Geometry: see drawing. Coordinates: mm, zero at the bounding-box minimum. Round coordinates to 2 decimals unless told otherwise and drop trailing zeros. Loops run counter-clockwise (first coordinate to the right, second up) from the corner with the lowest first, then second, coordinate; pieces in that order, holes last.
(1) Section C-C, the plane y = 14.5. Return the cut outline in (x, z), plus the area to 3 significant figures.
(2) Section A-A, the plane x = 33.5. Return the cut outline in (y, z).
(3) Section B-B, the plane z = 33.5. Return the cut outline in (x, y), plus the area to 3 significant figures.
(4) Material intervals for probe 1 along Z at (x, y) = (33.5, 17.75); probe 2 along Z at (x, y) = (45, 17); probe 3 along X at (y, z) = (18.75, 16.5), sorted ascending.
(5) Mould query, pull axis Z, two halves, no side actions, for the marked faces 1 and 2. Classes: pulls with the +Z half, pulls with the -Z half, needs draft (parallel to the pull), parting line crosses it, or undercut.
(6) First-contact query: pin 1 Ø6 at (y, z) = (7, 51.5) entering from -X; pin 2 Ø5 at (y, z) = (14.5, 43) entering from +X; pin 3 Ø8 at (x, y) = (18, 14.5) entering from -Z. Flat tips, straight axial feed; report the tip coordinate or a pass-through.
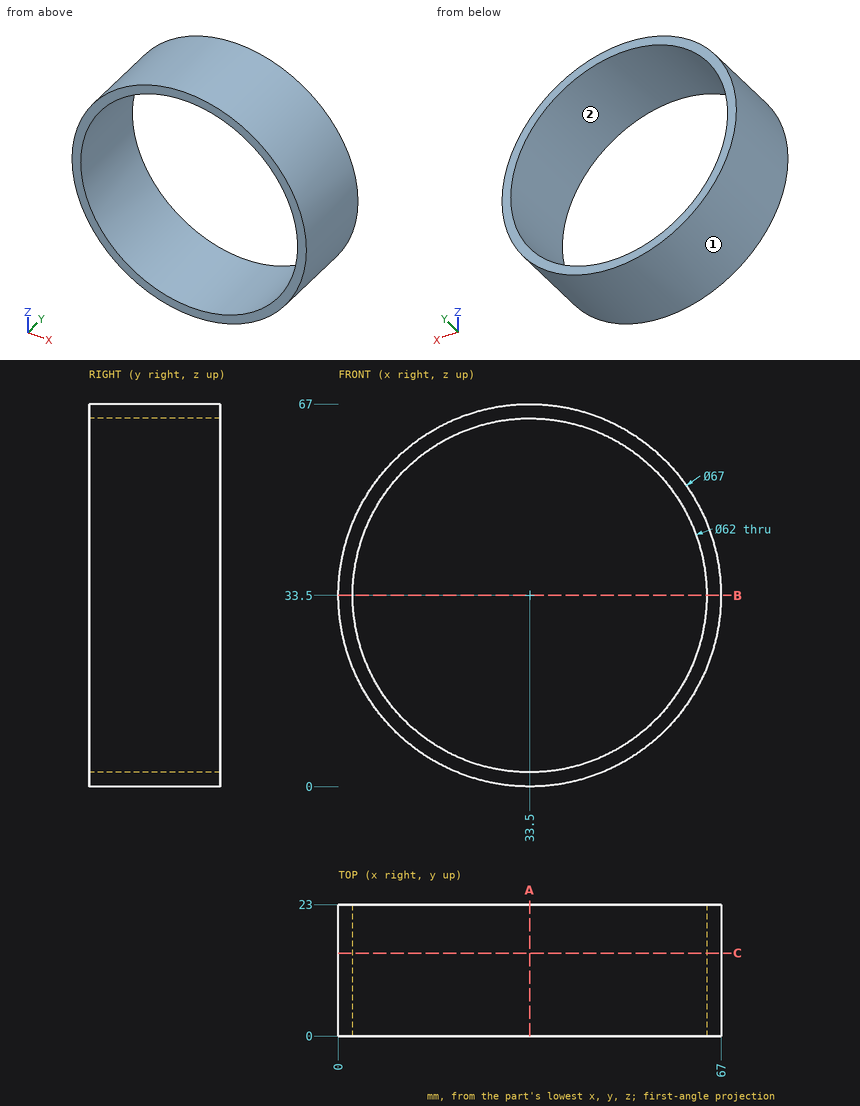
Output values:
1. outline: circle Ø67 at (33.5, 33.5); hole circle Ø62 at (33.5, 33.5)
1. area: 507 mm2
2. outline: (0, 0) - (23, 0) - (23, 2.5) - (0, 2.5) - close; (0, 64.5) - (23, 64.5) - (23, 67) - (0, 67) - close
3. outline: (0, 0) - (2.5, 0) - (2.5, 23) - (0, 23) - close; (64.5, 0) - (67, 0) - (67, 23) - (64.5, 23) - close
3. area: 115 mm2
4. probe 1: z = 0 to 2.5, 64.5 to 67
4. probe 2: z = 2.04 to 4.71, 62.29 to 64.96
4. probe 3: x = 4.63 to 7.58, 59.42 to 62.37
5. face 1: parting line crosses it
5. face 2: undercut
6. pin 1: stops at x = 3.55
6. pin 2: stops at x = 66.26
6. pin 3: stops at z = 2.04
